Work out the finished part from the listing and answer in its coordinate system (mm). Coordinates: 2 decimals unless noted, no trailing zeros. Loops run counter-clockwise (first coordinate to the right, second up) from the corner with the lowest first, then second, coordinate; pieces in that order, holes last. Notation, with made-up numbers: (-22, 76.25) - (-9, 76.25) arc R22 cw to (-9, 89.25) - close; hole circle Ø5 at (14, -29). An arc over 180 degrees is marked (long way). Write each question's results on one line, items separated by ' | '. Start each with the question number.
Item 1: Consider probe 1 along Y at (x, z) = (23.5, 5); probe 2 along X at (y, z) = (12.5, 7); probe 3 along X at (y, z) = (-3, 9.75). Determine where each line is inside the solid, lowest interval first. Write a range as [from, to].
Item 2: Section B-B, the plane z = 6.75 is taken. Count the separate pieces of the cut face and the enclosed holes in it, plus the area to 3 significant figures.
Item 3: Section D-D, the plane y = 34 is taken. Write down the section's boundary in (x, z), plus the area to 3 significant figures.
Item 4: Section C-C, the plane x = -45 is taken. Write down the section's boundary in (y, z), plus the area to 3 significant figures.
Item 5: For a pull along Y with two mould halves and no side action, classify faces 1 (the face through (-3, -40, 6)), 2 (the face through (-3, 18, 12)), 3 (the face through (42.79, 36.03, 6.08)) as +Y half, -Y half, draft (parallel to the pull), parting line (faces both ways), or undercut.
Item 6: Section A-A, the plane y = -10.5 is taken. Write down the section's boundary in (x, z).
from build123d import *

# Parameters (mm, degrees)
SKETCH1_W           = 360
SKETCH1_H           = 80
BOSS_EXTRUDE1_DEPTH = 12
CUT_EXTRUDE1_REACH  = 186.781
SKETCH2_R           = 3
SKETCH2_R_2         = 5
LPATTERN1_COUNT     = 4
LPATTERN1_PITCH     = 90
CUT_EXTRUDE2_REACH  = 186.781
SKETCH3_R           = 20
CUT_EXTRUDE3_REACH  = 186.781
SKETCH4_R           = 2


with BuildPart() as part:
    # Sketch1 → Boss-Extrude1 (new body)
    with BuildSketch(Plane.XY):
        Rectangle(SKETCH1_W, SKETCH1_H)
    extrude(amount=BOSS_EXTRUDE1_DEPTH)

    # Sketch2 → Cut-Extrude1 (cut, up to next)
    with BuildSketch(Plane.XY.offset(12), mode=Mode.PRIVATE) as cut_extrude1_sk1:
        with Locations((135, 34)):
            Circle(SKETCH2_R)
    cut_extrude1_tool1 = extrude(cut_extrude1_sk1.sketch, amount=-CUT_EXTRUDE1_REACH, mode=Mode.PRIVATE) & part.part
    # Sketch2 → Cut-Extrude1 (cut, up to next)
    with BuildSketch(Plane.XY.offset(12), mode=Mode.PRIVATE) as cut_extrude1_sk2:
        with Locations((135, -28)):
            Circle(SKETCH2_R_2)
    cut_extrude1_tool2 = extrude(cut_extrude1_sk2.sketch, amount=-CUT_EXTRUDE1_REACH, mode=Mode.PRIVATE) & part.part
    cut_extrude1_1 = cut_extrude1_tool1.solids().sort_by_distance((135, 34, 12))[0]
    add(cut_extrude1_1, mode=Mode.SUBTRACT)
    cut_extrude1_2 = cut_extrude1_tool2.solids().sort_by_distance((135, -28, 12))[0]
    add(cut_extrude1_2, mode=Mode.SUBTRACT)
    cut_extrude1 = cut_extrude1_1 + cut_extrude1_2  # Cut-Extrude1 as one shape, for the pattern or mirror that repeats it

    # LPattern1: Cut-Extrude1 ×4
    with Locations(*[(-i * LPATTERN1_PITCH, 0, 0) for i in range(1, LPATTERN1_COUNT)]):
        add(cut_extrude1, mode=Mode.SUBTRACT)

    # Sketch3 → Cut-Extrude2 (cut, up to next)
    with BuildSketch(Plane.XY.offset(12), mode=Mode.PRIVATE) as cut_extrude2_sk1:
        with Locations((0, -10.5)):
            Circle(SKETCH3_R)
    cut_extrude2_tool1 = extrude(cut_extrude2_sk1.sketch, amount=-CUT_EXTRUDE2_REACH, mode=Mode.PRIVATE) & part.part
    add(cut_extrude2_tool1.solids().sort_by_distance((0, -10.5, 12))[0], mode=Mode.SUBTRACT)

    # Sketch4 → Cut-Extrude3 (cut, up to next)
    with BuildSketch(Plane.XY.offset(12), mode=Mode.PRIVATE) as cut_extrude3_sk1:
        with Locations((-23.5, 13)):
            Circle(SKETCH4_R)
    cut_extrude3_tool1 = extrude(cut_extrude3_sk1.sketch, amount=-CUT_EXTRUDE3_REACH, mode=Mode.PRIVATE) & part.part
    # Sketch4 → Cut-Extrude3 (cut, up to next)
    with BuildSketch(Plane.XY.offset(12), mode=Mode.PRIVATE) as cut_extrude3_sk2:
        with Locations((-23.5, -34)):
            Circle(SKETCH4_R)
    cut_extrude3_tool2 = extrude(cut_extrude3_sk2.sketch, amount=-CUT_EXTRUDE3_REACH, mode=Mode.PRIVATE) & part.part
    cut_extrude3_1 = cut_extrude3_tool1.solids().sort_by_distance((-23.5, 13, 12))[0]
    add(cut_extrude3_1, mode=Mode.SUBTRACT)
    cut_extrude3_2 = cut_extrude3_tool2.solids().sort_by_distance((-23.5, -34, 12))[0]
    add(cut_extrude3_2, mode=Mode.SUBTRACT)
    cut_extrude3 = cut_extrude3_1 + cut_extrude3_2  # Cut-Extrude3 as one shape, for the pattern or mirror that repeats it

    # Mirror2: Cut-Extrude3 across plane
    add(cut_extrude3.mirror(Plane(origin=(0, 0, 0), x_dir=(0, 0, 1), z_dir=(1, 0, 0))), mode=Mode.SUBTRACT)


solid = part.part
Answer key:
1) probe 1: y = [-40, -36], [-32, 11], [15, 40] | probe 2: x = [-180, -25.44], [-21.56, 21.56], [25.44, 180] | probe 3: x = [-180, -18.54], [18.54, 180]
2) separate pieces: 1 | enclosed holes: 13 | area: 27,100 mm^2
3) outline: (-180, 0) - (-138, 0) - (-138, 12) - (-180, 12) - close; (-132, 0) - (-48, 0) - (-48, 12) - (-132, 12) - close; (-42, 0) - (42, 0) - (42, 12) - (-42, 12) - close; (48, 0) - (132, 0) - (132, 12) - (48, 12) - close; (138, 0) - (180, 0) - (180, 12) - (138, 12) - close | area: 4,030 mm^2
4) outline: (-40, 0) - (-33, 0) - (-33, 12) - (-40, 12) - close; (-23, 0) - (31, 0) - (31, 12) - (-23, 12) - close; (37, 0) - (40, 0) - (40, 12) - (37, 12) - close | area: 768 mm^2
5) face 1: -Y half | face 2: draft | face 3: undercut
6) outline: (-180, 0) - (-20, 0) - (-20, 12) - (-180, 12) - close; (20, 0) - (180, 0) - (180, 12) - (20, 12) - close
